Input: part model. Units: mm. Frame: model coordinates. Face numbers are marked on the shaded views. A direction names the side the tool comes from. Coordinates: 2 decimals unless noted, no trailing zeros. Order: outer loops, then holes, each group sorted by start corner. A loop starts at its lowest first (then second) coordinate and runs counter-clockwise, first axis right, second up. Notation, with made-up numbers: (-35, 37) -> (22, 37) arc R14 ccw to (22, 52) -> close; hole circle Ø7 at (88.5, -34.5). An arc over 180 degrees is marked (long way). Write each question's results on one line, items separated by ' | '.
```python
from build123d import *

# Parameters (mm, degrees)
SKETCH6_R      = 2.5
SKETCH6_W      = 20
SKETCH6_H      = 3
REVOLVE3_ANGLE = 270
SKETCH6_3_W    = 20
SKETCH6_3_H    = 3
REVOLVE4_ANGLE = 180
CHAMFER1_SIZE  = 5
FILLET1_R      = 2


with BuildPart() as part:
    # Sketch6 → Revolve3 (revolve)
    # profile 1 of 2: a face of its own
    with BuildSketch(Plane(origin=(0, 0, 0), x_dir=(0, 0, -1), z_dir=(1, 0, 0))):
        Polygon((20, 8), (20, 11), (20, 20), (0, 20), (0, 8), align=None)
        with Locations((10, 14)):
            Circle(SKETCH6_R, mode=Mode.SUBTRACT)
    # profile 2 of 2: a face of its own
    with BuildSketch(Plane(origin=(0, 0, 0), x_dir=(0, 0, -1), z_dir=(1, 0, 0))):
        with Locations((50, 9.5)):
            Rectangle(SKETCH6_W, SKETCH6_H)
    revolve(axis=Axis((0, 0, 0), (0, 0, 1)), revolution_arc=REVOLVE3_ANGLE)

    # Sketch6_3 → Revolve4 (revolve)
    with BuildSketch(Plane(origin=(0, 0, 0), x_dir=(0, 0, -1), z_dir=(1, 0, 0))):
        with Locations((30, 9.5)):
            Rectangle(SKETCH6_3_W, SKETCH6_3_H)
        with Locations((50, 9.5)):
            Rectangle(SKETCH6_3_W, SKETCH6_3_H)
    revolve(axis=Axis((0, 0, 0), (0, 0, 1)), revolution_arc=REVOLVE4_ANGLE)

    # Chamfer1
    chamfer1_edges = [part.edges().sort_by_distance(p)[0] for p in [
        (-5.656854249, -5.656854249, 0),
    ]]
    chamfer(chamfer1_edges, length=CHAMFER1_SIZE)

    # Fillet1
    fillet1_edges = [part.edges().sort_by_distance(p)[0] for p in [
        (-14.142135624, -14.142135624, 0),
    ]]
    fillet(fillet1_edges, radius=FILLET1_R)


solid = part.part
```
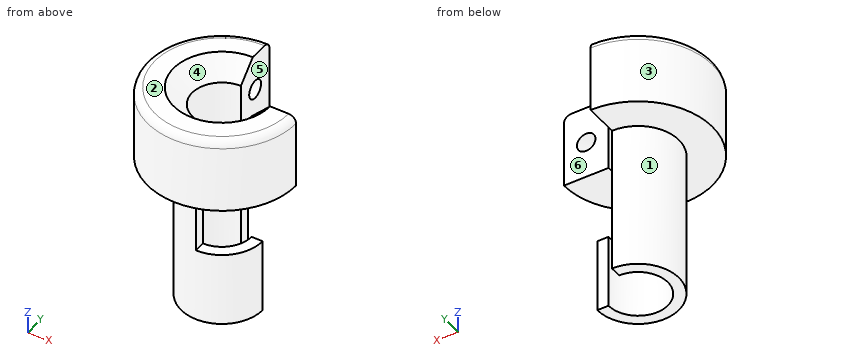
(1) Pin query (flat end, axial travel): P1, Ø1.5, axis at y = -9.5, z = -29.5, coming from the +X side; P2, Ø2.5, axis at x = 10, z = -45.5, coming from the +Y side; P3, Ø1.5, axis at y = -3.5, z = -52.5, coming from the +X side. Return the tip coordinate at first contact, or that it passes through.
Return value:
P1: x = 0 | P2: y = 0 | P3: x = 10.65
(2) Cut plane A-A, the plane x = 3.5. Count the separate pieces of the cut face and the enclosed holes in it, plus the area to 3 significant figures.
Return value:
separate pieces: 2 | enclosed holes: 1 | area: 280 mm2
(3) Line query: line 1 along Z through (x, y) = (-7.5, 12); line 2 along X through (y, z) = (0, -38); line 3 along X through (y, z) = (-3, -8). Output: solid intervals per line, ascending. Write a range as from..to.
Return value:
line 1: -20..-12.5, -7.5..0 | line 2: -11..-8 | line 3: -19.77..-15.21, -12.13..-7.42, 7.42..12.13, 15.21..19.77
(4) Reachability of the marked faces 1 and 2 from +Z, -Z, +X, -X, +Y, -Y: full face, straight path, thin tool, end or side. Return the list, or none.
Return value:
face 1: -Z | face 2: +Z, +X, -X, +Y, -Y
(5) Cut plane C-C, the plane z = -35.5. Return loops of the section in (x, y).
Return value:
outline: (0, -11) -> (0, -8) arc R8 cw to (0, 8) -> (0, 11) arc R11 ccw to start
(6) Mould query, pull axis X, two halves, no side actions, for the marked faces 3, 4, 5 and 6. Classes: +X half, -X half, draft (parallel to the pull), parting line (faces both ways), or undercut.
Return value:
face 3: parting line | face 4: undercut | face 5: +X half | face 6: draft
